The listing builds one solid part. Answer for the finished solid, in the listing's coordinates (mm). Round coordinates to 2 decimals unless told otherwise and drop trailing zeros. Order: outer loops, then holes, each group sorted by start corner. A loop starts at its lowest first (then second) coordinate and runs counter-clockwise, first axis right, second up. Notation, with made-up numbers: (86.5, 20.25) - (113.5, 20.25) arc R8 cw to (113.5, 34.25) - close; hole circle Ø5 at (9.25, 14). An arc over 180 degrees is marked (long way). Write item = value, one per line.
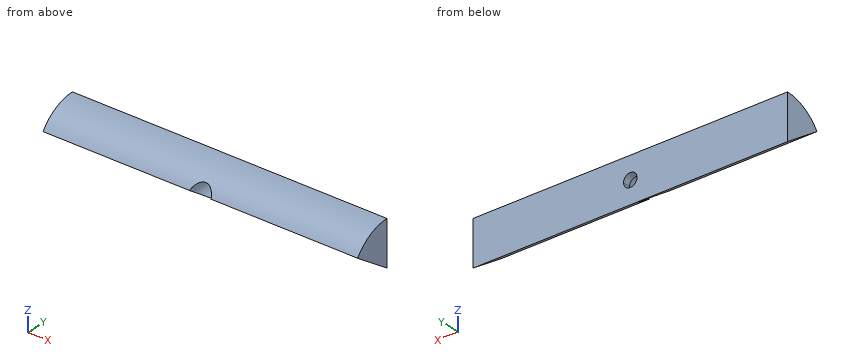
from build123d import *

# Parameters (mm, degrees)
F0_W     = 177.8
F0_H     = 25.4
F1_ANGLE = 55
F3_DEPTH = 20.8074619249
F5_R     = 6.35
F6_DEPTH = 16.51


with BuildPart() as f1:
    # F0 (on Front) → F1 (revolve)
    with BuildSketch(Plane.XZ):
        with Locations((88.9, 12.7)):
            Rectangle(F0_W, F0_H)
    revolve(axis=Axis((88.9, 0, 0), (1, 0, 0)), revolution_arc=F1_ANGLE)

    # F2 (on Front) → F3 (cut, through all)
    with BuildSketch(Plane.XZ):
        with BuildLine():
            ThreePointArc((88.9, 8.89), (91.5940768363, 10.0059231637), (92.71, 12.7))
            ThreePointArc((92.71, 12.7), (86.2059231637, 15.3940768363), (88.9, 8.89))
        make_face()
    extrude(amount=F3_DEPTH, mode=Mode.SUBTRACT)

    # F5 (on plane+point) → F6 (cut)
    with BuildSketch(Plane.XZ.offset(20.8064619249)):
        with Locations((88.9, 12.7)):
            Circle(F5_R)
    extrude(amount=-F6_DEPTH, mode=Mode.SUBTRACT)


solid = f1.part
Q1. Flat-ended cylindrical pins translate along their axes: P1, Ø10, axis at x = 21.5, y = -6.5, coming from the -Z side; P2, Ø1, axis at x = 116.5, y = -12, coming from the -Z side; P3, Ø10, axis at x = 88.9, z = 12.7, coming from the -Y side. Find the tip coordinate at first contact, or state that the pin passes through.
Model answer:
P1 = 1.05
P2 = 8.05
P3 = -4.3
Q2. Section B-B on y = -9 is taken. Determine the outline of the cut face in (x, z), then the cut area to 3 significant figures.
Model answer:
outline = (0, 6.3) - (177.8, 6.3) - (177.8, 23.75) - (0, 23.75) - close; hole circle Ø12.7 at (88.9, 12.7)
area = 2,980 mm^2
Q3. Section A-A on x = 91 is taken. Determine the outline of the cut face in (y, z), then the cut area to 3 significant figures.
Model answer:
outline = (-17.2, 18.69) - (-4.3, 18.69) - (-4.3, 15.88) - (0, 15.88) - (0, 25.4) arc R25.4 ccw to start; (-9.58, 6.71) - (0, 0) - (0, 9.52) - (-4.3, 9.52) - (-4.3, 6.71) - close
area = 135 mm^2
Q4. Section C-C on z = 3 is taken. Determine the outline of the cut face in (x, y).
Model answer:
outline = (0, -4.28) - (177.8, -4.28) - (177.8, 0) - (0, 0) - close
Q5. Find the intervals of material crossed by line 1 (X direction, y = -10.25, z = 12.7); line 2 (X direction, y = -1.1, z = 12.7); line 3 (Z direction, x = 88.9, y = -2), in increasing order. Write a range as from..to.
Model answer:
line_1 = 0..82.55, 95.25..177.8
line_2 = 0..85.09, 92.71..177.8
line_3 = 1.4..8.89, 16.51..25.32
